Input: part model. Units: mm. Frame: model coordinates. A direction names the side the tool comes from. Give positions to 0.01 mm unless a question says otherwise; leave off trailing zeros. Loops run counter-clockwise (first coordinate to the right, second up) from the corner with the lowest first, then second, coordinate; pieces in that order, holes last. Notation, with made-up numbers: (58, -18.5) - (78, -18.5) arc R26 cw to (78, 8.5) - close; hole circle Ø2 at (36, 45). An arc over 180 degrees is marked (long way). Answer as a JSON object with one key per item and string values.
from build123d import *

# Parameters (mm, degrees)
MODEL_R                 = 27
MODEL_R_2               = 2
MODEL_R_3               = 3.5
MODEL_R_4               = 1.5
SALIENTE_EXTRUIR1_DEPTH = 3
CROQUIS2_W              = 6.5
CROQUIS2_H              = 6.5
CORTAR_EXTRUIR1_DEPTH   = 2


with BuildPart() as part:
    # Model → Saliente-Extruir1 (new body)
    with BuildSketch(Plane.XY):
        with Locations((216.74059699, 240.760681356)):
            Circle(MODEL_R)
        with Locations((216.74059699, 240.760681356)):
            Circle(MODEL_R_2, mode=Mode.SUBTRACT)
        with Locations((216.74059699, 260.885293153)):
            Circle(MODEL_R_3, mode=Mode.SUBTRACT)
        with Locations((216.74059699, 249.760681356)):
            Circle(MODEL_R_4, mode=Mode.SUBTRACT)
        with Locations((234.169022048, 250.822987255)):
            Circle(MODEL_R_3, mode=Mode.SUBTRACT)
        with Locations((234.169022048, 230.698375457)):
            Circle(MODEL_R_3, mode=Mode.SUBTRACT)
        with Locations((216.74059699, 231.760681356)):
            Circle(MODEL_R_4, mode=Mode.SUBTRACT)
        with Locations((216.74059699, 220.636069558)):
            Circle(MODEL_R_3, mode=Mode.SUBTRACT)
        with Locations((199.312171932, 230.698375457)):
            Circle(MODEL_R_3, mode=Mode.SUBTRACT)
        with Locations((199.312171932, 250.822987255)):
            Circle(MODEL_R_3, mode=Mode.SUBTRACT)
        with BuildLine():
            Line((210.36559699, 244.010681356), (212.11559699, 244.010681356))
            ThreePointArc((212.11559699, 244.010681356), (212.645927076, 243.791011442), (212.86559699, 243.260681356))
            Line((212.86559699, 243.260681356), (212.86559699, 238.260681356))
            ThreePointArc((212.86559699, 238.260681356), (212.645927076, 237.73035127), (212.11559699, 237.510681356))
            Line((212.11559699, 237.510681356), (210.36559699, 237.510681356))
            ThreePointArc((210.36559699, 237.510681356), (209.835266904, 237.73035127), (209.61559699, 238.260681356))
            Line((209.61559699, 238.260681356), (209.61559699, 243.260681356))
            ThreePointArc((209.61559699, 243.260681356), (209.835266904, 243.791011442), (210.36559699, 244.010681356))
        make_face(mode=Mode.SUBTRACT)
        with BuildLine():
            Line((223.11559699, 244.010681356), (221.36559699, 244.010681356))
            ThreePointArc((221.36559699, 244.010681356), (220.835266904, 243.791011442), (220.61559699, 243.260681356))
            Line((220.61559699, 243.260681356), (220.61559699, 238.260681356))
            ThreePointArc((220.61559699, 238.260681356), (220.835266904, 237.73035127), (221.36559699, 237.510681356))
            Line((221.36559699, 237.510681356), (223.11559699, 237.510681356))
            ThreePointArc((223.11559699, 237.510681356), (223.645927076, 237.73035127), (223.86559699, 238.260681356))
            Line((223.86559699, 238.260681356), (223.86559699, 243.260681356))
            ThreePointArc((223.86559699, 243.260681356), (223.645927076, 243.791011442), (223.11559699, 244.010681356))
        make_face(mode=Mode.SUBTRACT)
        with BuildLine():
            Line((226.523367563, 226.246291995), (228.061081049, 227.143741747))
            ThreePointArc((228.061081049, 227.143741747), (230.275423122, 226.529484608), (229.661165983, 224.315142535))
            Line((229.661165983, 224.315142535), (227.185628981, 222.869606716))
            ThreePointArc((227.185628981, 222.869606716), (226.586226063, 222.662900739), (225.953347023, 222.701310884))
            Line((225.953347023, 222.701310884), (221.3946266, 224.629068514))
            ThreePointArc((221.3946266, 224.629068514), (220.652146842, 226.65572191), (222.577128703, 227.631962152))
            Line((222.577128703, 227.631962152), (225.84390332, 226.242471741))
            ThreePointArc((225.84390332, 226.242471741), (226.184030387, 226.174137605), (226.523367563, 226.246291995))
        make_face(mode=Mode.SUBTRACT)
        with BuildLine():
            Line((234.201812184, 241.975614511), (234.193454642, 243.75603833))
            ThreePointArc((234.193454642, 243.75603833), (235.832587966, 245.366586248), (237.443135884, 243.727452924))
            Line((237.443135884, 243.727452924), (237.457238125, 240.860807084))
            ThreePointArc((237.457238125, 240.860807084), (237.336549293, 240.238355941), (236.986845611, 239.709471687))
            Line((236.986845611, 239.709471687), (233.03799832, 236.725382808))
            ThreePointArc((233.03799832, 236.725382808), (230.911625115, 237.095703172), (231.028667196, 239.250906488))
            Line((231.028667196, 239.250906488), (233.865388499, 241.385271088))
            ThreePointArc((233.865388499, 241.385271088), (234.09463113, 241.6456627), (234.201812184, 241.975614511))
        make_face(mode=Mode.SUBTRACT)
        with BuildLine():
            Line((224.41904161, 256.490003872), (222.872970584, 257.372977938))
            ThreePointArc((222.872970584, 257.372977938), (222.297761834, 259.597782996), (224.522566892, 260.172991745))
            Line((224.522566892, 260.172991745), (227.012206134, 258.751881723))
            ThreePointArc((227.012206134, 258.751881723), (227.49092022, 258.336136558), (227.774095579, 257.768842159))
            Line((227.774095579, 257.768842159), (228.38396871, 252.856995649))
            ThreePointArc((228.38396871, 252.856995649), (227.000075264, 251.200662618), (225.192135483, 252.379625691))
            Line((225.192135483, 252.379625691), (224.76208217, 255.903480703))
            ThreePointArc((224.76208217, 255.903480703), (224.651197734, 256.232206452), (224.41904161, 256.490003872))
        make_face(mode=Mode.SUBTRACT)
        with BuildLine():
            Line((199.279381797, 239.5457482), (199.287739338, 237.765324382))
            ThreePointArc((199.287739338, 237.765324382), (197.648606014, 236.154776464), (196.038058096, 237.793909788))
            Line((196.038058096, 237.793909788), (196.023955856, 240.660555628))
            ThreePointArc((196.023955856, 240.660555628), (196.144644688, 241.283006771), (196.494348369, 241.811891025))
            Line((196.494348369, 241.811891025), (200.44319566, 244.795979904))
            ThreePointArc((200.44319566, 244.795979904), (202.569568865, 244.42565954), (202.452526784, 242.270456224))
            Line((202.452526784, 242.270456224), (199.615805481, 240.136091624))
            ThreePointArc((199.615805481, 240.136091624), (199.38656285, 239.875700011), (199.279381797, 239.5457482))
        make_face(mode=Mode.SUBTRACT)
        with BuildLine():
            Line((209.06215237, 225.03135884), (210.608223397, 224.148384774))
            ThreePointArc((210.608223397, 224.148384774), (211.183432146, 221.923579716), (208.958627088, 221.348370966))
            Line((208.958627088, 221.348370966), (206.468987847, 222.769480989))
            ThreePointArc((206.468987847, 222.769480989), (205.990273761, 223.185226154), (205.707098402, 223.752520553))
            Line((205.707098402, 223.752520553), (205.097225271, 228.664367063))
            ThreePointArc((205.097225271, 228.664367063), (206.481118716, 230.320700093), (208.289058497, 229.141737021))
            Line((208.289058497, 229.141737021), (208.719111811, 225.617882009))
            ThreePointArc((208.719111811, 225.617882009), (208.829996246, 225.28915626), (209.06215237, 225.03135884))
        make_face(mode=Mode.SUBTRACT)
        with BuildLine():
            Line((206.957826417, 255.275070717), (205.420112932, 254.377620965))
            ThreePointArc((205.420112932, 254.377620965), (203.205770858, 254.991878104), (203.820027998, 257.206220177))
            Line((203.820027998, 257.206220177), (206.295564999, 258.651755995))
            ThreePointArc((206.295564999, 258.651755995), (206.894967917, 258.858461972), (207.527846958, 258.820051828))
            Line((207.527846958, 258.820051828), (212.08656738, 256.892294198))
            ThreePointArc((212.08656738, 256.892294198), (212.829047139, 254.865640802), (210.904065277, 253.889400559))
            Line((210.904065277, 253.889400559), (207.637290661, 255.278890971))
            ThreePointArc((207.637290661, 255.278890971), (207.297163594, 255.347225107), (206.957826417, 255.275070717))
        make_face(mode=Mode.SUBTRACT)
    extrude(amount=SALIENTE_EXTRUIR1_DEPTH)

    # Croquis2 → Cortar-Extruir1 (cut)
    with BuildSketch(Plane.XY.offset(3)):
        with Locations((216.74059699, 249.760681356)):
            Rectangle(CROQUIS2_W, CROQUIS2_H)
        with Locations((216.74059699, 231.760681356)):
            Rectangle(CROQUIS2_W, CROQUIS2_H)
    extrude(amount=-CORTAR_EXTRUIR1_DEPTH, mode=Mode.SUBTRACT)


solid = part.part
Item 1: Material intervals for line 1 (X direction, y = 232, z = 1.6); line 2 (Y direction, x = 218.5, z = 1.7); line 3 (Y direction, x = 215, z = 1.75), sorted ascending. Write a range as [from, to].
Geometry check:
{"line 1": "x = [191.2, 196.06], [202.56, 213.49], [219.99, 230.92], [237.42, 242.28]", "line 2": "y = [213.82, 217.61], [223.66, 228.51], [235.01, 239.81], [241.71, 246.51], [253.01, 257.86], [263.91, 267.7]", "line 3": "y = [213.82, 217.6], [223.67, 228.51], [235.01, 239.78], [241.75, 246.51], [253.01, 257.85], [263.92, 267.7]"}
Item 2: Cut plane A-A (x = 198). Return loops of the section in (y, z), then the cut area to 3 significant figures.
Geometry check:
{"outline": "(221.32, 0) - (227.45, 0) - (227.45, 3) - (221.32, 3) - close; (233.94, 0) - (236.19, 0) - (236.19, 3) - (233.94, 3) - close; (242.95, 0) - (247.58, 0) - (247.58, 3) - (242.95, 3) - close; (254.07, 0) - (260.2, 0) - (260.2, 3) - (254.07, 3) - close", "area": "57.4 mm2"}
Item 3: Contact query for flat-ended pins moving along their axis: P1, Ø1, axis at x = 211.5, z = 2, coming from the -Y side; P2, Ø1, axis at x = 218.5, z = 2.5, coming from the -Y side; P3, Ø1, axis at y = 250.5, z = 1.5, coming from the +X side. Output: stop coordinate, or through.
Geometry check:
{"P1": "stops at y = 214.18", "P2": "stops at y = 213.79", "P3": "stops at x = 242.11"}
Item 4: Cut plane B-B (y = 261.5). Return loops of the section in (x, z) (3 decimals).
Geometry check:
{"outline": "(199.452, 0) - (213.295, 0) - (213.295, 3) - (199.452, 3) - close; (220.186, 0) - (234.029, 0) - (234.029, 3) - (220.186, 3) - close"}
Item 5: Cut plane C-C (z = 1.7). Give the number of separate pieces and of enclosed holes in the cut face, then the cut area to 3 significant figures.
Geometry check:
{"separate pieces": "1", "enclosed holes": "17", "area": "1,730 mm2"}
Item 6: Access query for faces 1 (the face through (206.2, 254.833, 1.479)), 2 (the face through (217, 235.011, 2)). Directions: +Z, -Z, +X, -X, +Y, -Y. A direction counts if a zero-diameter tool reaches every point of the face in a straight line with its end or side. Return the directions, or none.
Geometry check:
{"face 1": "+Z, -Z", "face 2": "+Z"}
